```python
from build123d import *

# Parameters (mm, degrees)
ESQUISSE1_W             = 65
ESQUISSE1_H             = 65
BOSS_EXTRU_1_DEPTH      = 1
BOSS_EXTRU_2_START      = 1
BOSS_EXTRU_2_DEPTH      = 100
ENL_V_MAT_EXTRU_1_REACH = 161.619
CONG_1_R                = 7.5


with BuildPart() as part:
    # Esquisse1 → Boss.-Extru.1 (new body)
    with BuildSketch(Plane(origin=(0, 0, 0), x_dir=(1, 0, 0), z_dir=(0, 1, 0))):
        with Locations((75, 75)):
            Rectangle(ESQUISSE1_W, ESQUISSE1_H)
        with BuildLine():
            Line((47.5, 67.516685226), (47.5, 75))
            ThreePointArc((47.5, 75), (75, 102.5), (102.5, 75))
            Line((102.5, 75), (102.5, 67.516685226))
            ThreePointArc((102.5, 67.516685226), (75, 46.5), (47.5, 67.516685226))
        make_face(mode=Mode.SUBTRACT)
    extrude(amount=BOSS_EXTRU_1_DEPTH)

    # Esquisse1<3> → Boss.-Extru.2 (add)
    with BuildSketch(Plane(origin=(0, 0, 0), x_dir=(1, 0, 0), z_dir=(0, 1, 0)).offset(BOSS_EXTRU_2_START)):
        with BuildLine():
            ThreePointArc((103.5, 75), (75, 103.5), (46.5, 75))
            Line((46.5, 75), (46.5, 46.608370242))
            Line((46.5, 46.608370242), (47.5, 47.5))
            Line((47.5, 47.5), (47.5, 67.516685226))
            Line((47.5, 67.516685226), (47.5, 75))
            ThreePointArc((47.5, 75), (75, 102.5), (102.5, 75))
            Line((102.5, 75), (102.5, 67.516685226))
            Line((102.5, 67.516685226), (102.5, 47.5))
            Line((102.5, 47.5), (103.5, 46.608370242))
            Line((103.5, 46.608370242), (103.5, 75))
        make_face()
    extrude(amount=BOSS_EXTRU_2_DEPTH)

    # Enlèv. mat.-Extru.1: up to this face of the body (flat: up to its plane)
    enl_v_mat_extru_1_end = Plane(part.part.faces().sort_by_distance((103.5, 51, -60.804185121))[0])
    # Esquisse2 → Enlèv. mat.-Extru.1 (cut, up to the picked face)
    with BuildSketch(Plane.ZY.offset(-46.5), mode=Mode.PRIVATE) as enl_v_mat_extru_1_sk1:
        Polygon((-46.608370242, 1), (-75, 101), (-46.608370242, 101), align=None)
    enl_v_mat_extru_1_tool1 = split(extrude(enl_v_mat_extru_1_sk1.sketch, amount=-ENL_V_MAT_EXTRU_1_REACH, mode=Mode.PRIVATE), bisect_by=enl_v_mat_extru_1_end, keep=Keep.BOTH, mode=Mode.PRIVATE)
    add(enl_v_mat_extru_1_tool1.solids().sort_by(Axis((46.5, 67.666667, -56.072247), (1, 0, 0)))[0], mode=Mode.SUBTRACT)

    # Congé1
    cong_1_edges = [part.edges().sort_by_distance(p)[0] for p in [
        (42.5, 0.5, -42.5),
        (42.5, 0.5, -107.5),
        (107.5, 0.5, -107.5),
        (107.5, 0.5, -42.5),
    ]]
    fillet(cong_1_edges, radius=CONG_1_R)


solid = part.part
```
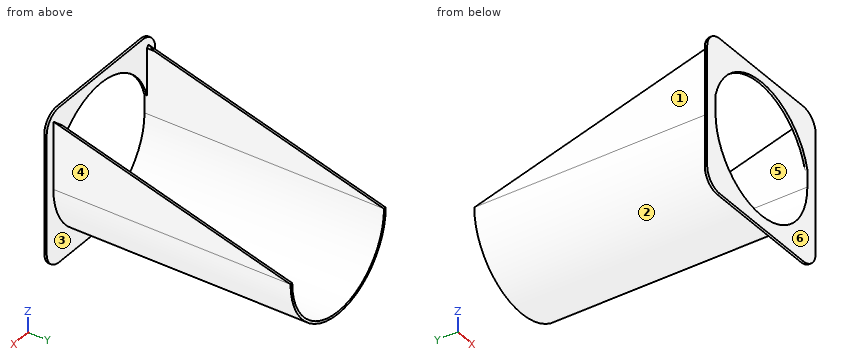
Read the model definition and answer for the solid it produces. Units are mm, in the model's axes. Face numbers are marked on the shaded views. A direction names the side the tool comes from. Give positions to 0.01 mm unless a question says otherwise; leave off trailing zeros. Order: outer loops, then holes, each group sorted by start corner. A loop starts at its lowest first (then second) coordinate and runs counter-clockwise, first axis right, second up. Notation, with made-up numbers: (3, 12) -> (48, 12) arc R20 cw to (48, 32) -> close; hole circle Ø2 at (48.5, 86). An arc over 180 degrees is marked (long way). One line per item, written item: value. Start each with the question number.
(1) The part is cut by section B-B (z = -93). Determine the outline of the cut face in (x, y).
(2) The part is cut by section D-D (x = 54). Determine the outline of the cut face in (y, z), and give its area (3 significant figures).
(3) A tool of negligible diameter and unlimited length cuts with its end or side. For the marked faces 1, 2 and 3, from which of +Z, -Z, +X, -X, +Y, -Y can it reach the whole face along a straight path? Write none if from no direction.
(4) The part is cut by section A-A (x = 75). Determine the outline of the cut face in (y, z), and give its area (3 significant figures).
(5) Straight lines are drawn through the part: L1, parallel to X at y = 42, z = -63; L2, parallel to Y at x = 50, z = -101.5; L3, parallel to X at y = 5, z = -91. For each, find the intervals that lie inside material, in ascending order.
(6) Flat-ended cylindrical pins translate along their axes: P1, Ø14, axis at y = 29.5, z = -68, coming from the +X side; P2, Ø6, axis at y = 68.5, z = -75.5, coming from the -X side; P3, Ø1, axis at y = 88, z = -87, coming from the +X side. Find the tip coordinate at first contact, or state that the pin passes through.
(7) For a pull along X with two mould halves and no side action, classify the marked faces 4, 5 and 6 as released by +X, released by -X, zero draft, split by the parting line, or undercut.
(8) The part is cut by section C-C (y = 62). Determine the outline of the cut face in (x, z), and give its area (3 significant figures).
Taken from the geometry:
1. outline: (42.5, 0) -> (54.21, 0) -> (54.21, 101) -> (52.9, 101) -> (52.9, 1) -> (42.5, 1) -> close; (95.79, 0) -> (107.5, 0) -> (107.5, 1) -> (97.1, 1) -> (97.1, 101) -> (95.79, 101) -> close
2. outline: (0, -107.5) -> (1, -107.5) -> (1, -94.27) -> (101, -94.27) -> (101, -92.76) -> (0, -92.76) -> close; (0, -55.73) -> (1, -55.73) -> (1, -42.5) -> (0, -42.5) -> close
2. area: 179 mm^2
3. face 1: +Z, -Z, -X, +Y
3. face 2: -Z, +Y
3. face 3: +Y
4. outline: (0, -107.5) -> (1, -107.5) -> (1, -103.5) -> (101, -103.5) -> (101, -102.5) -> (0, -102.5) -> close; (0, -46.5) -> (1, -46.5) -> (1, -42.5) -> (0, -42.5) -> close
4. area: 109 mm^2
5. L1: 46.5 to 47.5, 102.5 to 103.5
5. L2: 0 to 1
5. L3: 51.42 to 52.63, 97.37 to 98.58
6. P1: x = 103.5
6. P2: x = 46.5
6. P3: x = 101.08
7. face 4: released by +X
7. face 5: undercut
7. face 6: zero draft
8. outline: (46.5, -75) arc R28.5 ccw to (103.5, -75) -> (103.5, -63.93) -> (102.5, -63.93) -> (102.5, -75) arc R27.5 cw to (47.5, -75) -> (47.5, -63.93) -> (46.5, -63.93) -> close
8. area: 110 mm^2
